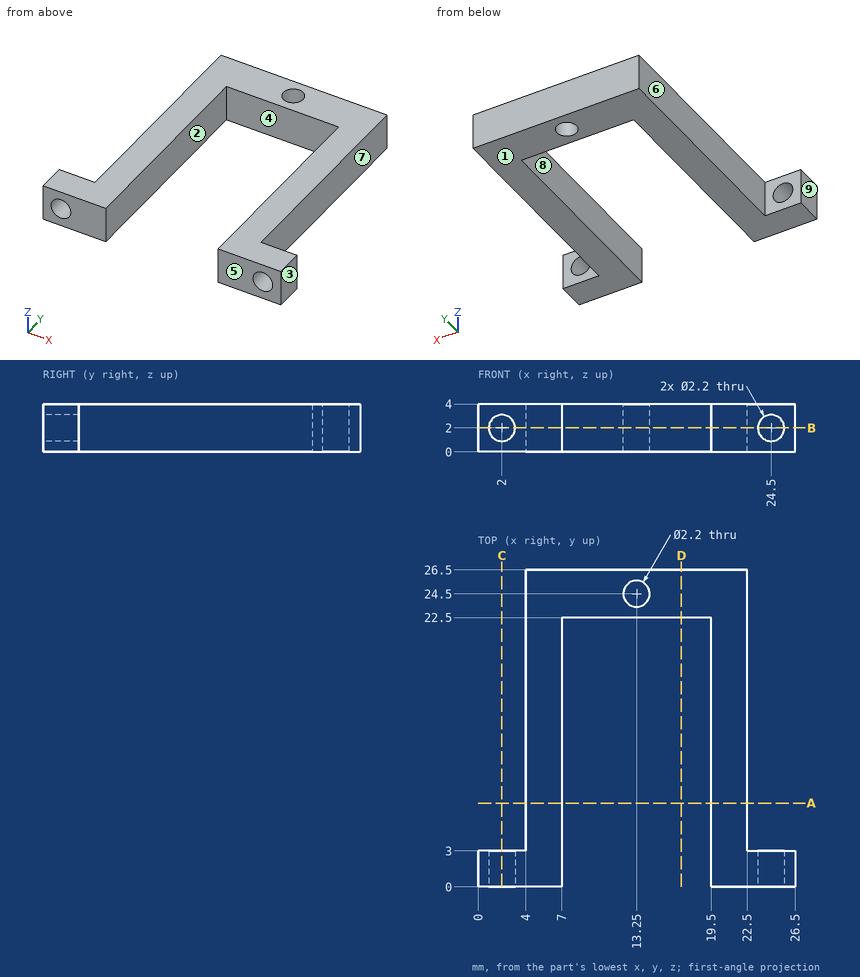
Can you work these out from the drawing? Everything is in mm from the part's minimum corner. A direction names the side the tool comes from. Round coordinates to 2 decimals unless told otherwise and drop trailing zeros. Order: outer loops, then holes, each group sorted by start corner. A loop starts at its lowest first (then second) coordinate and runs counter-clockwise, first axis right, second up. Notation, with made-up numbers: (58, 74) - (92, 74) arc R19 ccw to (92, 98) - close; hole circle Ø10 at (-25, -7.5). An arc over 180 degrees is marked (long way). Answer in a Markdown table with one row per item.
(1) For P1, Ø1.2, axis at x = 2.5, z = 1, coming from the +Y side; P2, Ø2, axis at y = 20, z = 2, coming from the -X side; P3, Ø2, axis at y = 15, z = 2, coming from the +X side, each with a flat end and sliding along its axis, tell me the tip position at first contact or that it passes through.
From the geometry:
| item | result |
|---|---|
| P1 | stops at y = 3 |
| P2 | stops at x = 4 |
| P3 | stops at x = 22.5 |
(2) Suppose I cut it at D-D, the plane x = 17. Please give me the cut outline in (y, z).
From the geometry:
| item | result |
|---|---|
| outline | (22.5, 0) - (26.5, 0) - (26.5, 4) - (22.5, 4) - close |
(3) If we mould it in two halves opening along X, with no side actions, what happens to the marked faces 1, 2, 3 and 4? For each: released by +X, released by -X, zero draft, split by the parting line, or undercut.
From the geometry:
| item | result |
|---|---|
| face 1 | zero draft |
| face 2 | undercut |
| face 3 | released by +X |
| face 4 | undercut |
(4) Suppose I cut it at B-B, the plane z = 2. Please give me the cut outline in (x, y), plus the area to 3 significant figures.
From the geometry:
| item | result |
|---|---|
| outline | (0, 0) - (0.9, 0) - (0.9, 3) - (0, 3) - close; (3.1, 0) - (7, 0) - (7, 22.5) - (19.5, 22.5) - (19.5, 0) - (23.4, 0) - (23.4, 3) - (22.5, 3) - (22.5, 26.5) - (4, 26.5) - (4, 3) - (3.1, 3) - close; (25.6, 0) - (26.5, 0) - (26.5, 3) - (25.6, 3) - close; hole circle Ø2.2 at (13.25, 24.5) |
| area | 216 mm2 |
(5) Suppose I cut it at A-A, the plane y = 7. Please give me the cut outline in (x, z).
From the geometry:
| item | result |
|---|---|
| outline | (4, 0) - (7, 0) - (7, 4) - (4, 4) - close; (19.5, 0) - (22.5, 0) - (22.5, 4) - (19.5, 4) - close |
(6) Suppose I cut it at C-C, the plane x = 2. Please give me the cut outline in (y, z).
From the geometry:
| item | result |
|---|---|
| outline | (0, 0) - (3, 0) - (3, 0.9) - (0, 0.9) - close; (0, 3.1) - (3, 3.1) - (3, 4) - (0, 4) - close |
(7) Please list where these lines run through material, in increasing order: L1, parallel to X at y = 1.65, z = 2; L2, parallel to X at y = 18.25, z = 3.4; L3, parallel to Z at x = 24.5, y = 0.85. Write a range as from..to.
From the geometry:
| item | result |
|---|---|
| L1 | x = 0..0.9, 3.1..7, 19.5..23.4, 25.6..26.5 |
| L2 | x = 4..7, 19.5..22.5 |
| L3 | z = 0..0.9, 3.1..4 |
(8) Which directions (+Z, -Z, +X, -X, +Y, -Y) give clear straight access to the entire face, cutting with the end or side of a thin tool? Please do the marked faces 5, 6, 7, 8 and 9.
From the geometry:
| item | result |
|---|---|
| face 5 | +Z, -Z, +X, -X, -Y |
| face 6 | +Z, -Z, -X, +Y |
| face 7 | +Z, -Z, +X, +Y |
| face 8 | +Z, -Z, -Y |
| face 9 | +Z, -Z, -X, +Y, -Y |
